```python
from build123d import *

# Parameters (mm, degrees)
SKETCH1_R           = 1.5875
SKETCH1_R_2         = 1.7859375
BOSS_EXTRUDE1_DEPTH = 1.5875
FILLET1_R           = 0.4064
FILLET2_R           = 3.571875


with BuildPart() as part:
    # Sketch1 → Boss-Extrude1 (new body)
    with BuildSketch(Plane.XY):
        with BuildLine():
            ThreePointArc((17.462464722, 10.31875), (14.287464722, 13.49375), (11.112464722, 10.31875))
            Line((11.112464722, 10.31875), (11.112464722, 5.55625))
            Line((11.112464722, 5.55625), (0, 5.55625))
            ThreePointArc((0, 5.55625), (-5.113201992, 2.17418478), (-4.001636336, -3.854714088))
            ThreePointArc((-4.001636336, -3.854714088), (-3.061446663, -5.6851033), (-3.287058398, -7.730434724))
            ThreePointArc((-3.287058398, -7.730434724), (-0.713207299, -12.628071623), (3.571875, -9.128125))
            ThreePointArc((3.571875, -9.128125), (4.61805296, -6.602427972), (7.143749984, -5.55625))
            Line((7.143749984, -5.55625), (12.699964722, -5.55625))
            Line((12.699964722, -5.55625), (12.699964722, -6.36905))
            Line((12.699964722, -6.36905), (15.874964722, -6.36905))
            Line((15.874964722, -6.36905), (15.874964722, -5.130880657))
            ThreePointArc((15.874964722, -5.130880657), (17.037095379, -3.96875), (17.462464722, -2.38125))
            Line((17.462464722, -2.38125), (17.462464722, 10.31875))
        make_face()
        with Locations((14.287464722, 0.03175)):
            Circle(SKETCH1_R, mode=Mode.SUBTRACT)
        with Locations((14.287464722, 7.90575)):
            Circle(SKETCH1_R, mode=Mode.SUBTRACT)
        Circle(SKETCH1_R_2, mode=Mode.SUBTRACT)
        with Locations((0, -9.128125)):
            Circle(SKETCH1_R_2, mode=Mode.SUBTRACT)
    extrude(amount=BOSS_EXTRUDE1_DEPTH)

    # Fillet1
    fillet1_edges = [part.edges().sort_by_distance(p)[0] for p in [
        (15.874964722, -5.130880657, 0.79375),
        (15.874964722, -6.36905, 0.79375),
        (12.699964722, -5.55625, 0.79375),
        (12.699964722, -6.36905, 0.79375),
    ]]
    fillet(fillet1_edges, radius=FILLET1_R - 0.0001)  # a hair under: the kernel refuses the full size

    # Fillet2
    fillet2_edges = [part.edges().sort_by_distance(p)[0] for p in [
        (11.112464722, 5.55625, 0.79375),
    ]]
    fillet(fillet2_edges, radius=FILLET2_R)


solid = part.part
```
CAD build for the part. Positions are in the model's coordinates, mm. A direction names the side the tool comes from. Round coordinates to 2 decimals unless told otherwise and drop trailing zeros. Answer in a Markdown table with one row per item. Add a question column.
Item 1: Drill centre lines: line 1 (Y direction, x = 1, z = 0.75); line 2 (Y direction, x = 13.25, z = 0.3); line 3 (X direction, y = 0.25, z = 0.8). Where is each one in solid material? Low to high. Write a range as from..to.
Item 2: Drop flat-ended pins along their axis: pin 1 Ø3 at (x, y) = (0, 0) entering from -Z; pin 2 Ø0.5 at (x, z) = (14.5, 1) entering from -Y; pin 3 Ø0.5 at (y, z) = (-6, 1) entering from +X; pin 4 Ø12 at (x, y) = (-3, -4.5) entering from -Z. Give the stop position or say it passes through.
Item 3: Mould opens along X. For faces 3 (the face through (10, -5.556, 1)), 4 (the face through (14, -6.369, 1)), 5 (the face through (14.357, 13.493, 0.783)) say: pulls with the +X half, pulls with the -X half, needs draft (parallel to the pull), parting line crosses it, or undercut.
Item 4: Which spindle directions (+Z, -Z, +X, -X, +Y, -Y) get a long thin tool onto all of the face, cutting with end or side? Do faces 1 (the face through (11.112, 10, 1)), 2 (the face through (6, 1, 0)). Say none if no direction does.
Item 5: Saw through at A-A, the plane z = 0.9. Count the separate pieces of the cut face and the enclosed holes in it, then the cut area to 3 significant figures.
Findings below:
| question | item | result |
|---|---|---|
| 1 | line 1 | y = -12.56..-10.61, -7.65..-1.48, 1.48..5.56 |
| 1 | line 2 | y = -6.37..-1.17, 1.23..6.7, 9.11..13.32 |
| 1 | line 3 | x = -5.55..-1.77, 1.77..12.72, 15.86..17.46 |
| 2 | pin 1 | passes through |
| 2 | pin 2 | stops at y = -6.37 |
| 2 | pin 3 | stops at x = 15.87 |
| 2 | pin 4 | stops at z = 0 |
| 3 | face 3 | undercut |
| 3 | face 4 | needs draft |
| 3 | face 5 | parting line crosses it |
| 4 | face 1 | +Z, -Z, -X, +Y |
| 4 | face 2 | -Z, +X, -X, +Y, -Y |
| 5 | separate pieces | 1 |
| 5 | enclosed holes | 4 |
| 5 | area | 304 mm^2 |
